```python
from build123d import *

# Parameters (mm, degrees)
F1_DEPTH = 25.4


with BuildPart() as f1:
    # F0 (on Top) → F1 (new body)
    with BuildSketch(Plane.XY):
        with BuildLine():
            ThreePointArc((0.5710253026, 3.1232283144), (0.8333744276, 3.0636762335), (1.0897403684, 2.9821285904))
            Line((1.0897403684, 2.9821285904), (1.0897403684, 10.6021285904))
            Line((1.0897403684, 10.6021285904), (0.5710253026, 10.6021285904))
            Line((0.5710253026, 10.6021285904), (0.5710253026, 3.1232283144))
        make_face()
        with BuildLine():
            ThreePointArc((-1.0897403684, 2.9821285904), (-0.8333744276, 3.0636762335), (-0.5710253026, 3.1232283144))
            Line((-0.5710253026, 3.1232283144), (-0.5710253026, 10.6021285904))
            Line((-0.5710253026, 10.6021285904), (-1.0897403684, 10.6021285904))
            Line((-1.0897403684, 10.6021285904), (-1.0897403684, 2.9821285904))
        make_face()
        with BuildLine():
            ThreePointArc((-2.9903077134, -1.0670917389), (-3.0699086609, -0.8101146916), (-3.1274693008, -0.5473214526))
            Line((-3.1274693008, -0.5473214526), (-9.7265828776, -4.3573214526))
            Line((-9.7265828776, -4.3573214526), (-9.4672253448, -4.8065418769))
            Line((-9.4672253448, -4.8065418769), (-2.9903077134, -1.0670917389))
        make_face()
        with BuildLine():
            Line((-8.6368425092, -6.2448071378), (-2.0377289324, -2.4348071378))
            ThreePointArc((-2.0377289324, -2.4348071378), (-2.2365342333, -2.2535615419), (-2.4192824108, -2.0561365755))
            Line((-2.4192824108, -2.0561365755), (-8.8962000421, -5.7955867135))
            Line((-8.8962000421, -5.7955867135), (-8.6368425092, -6.2448071378))
        make_face()
        with BuildLine():
            Line((8.8962000421, -5.7955867135), (2.4192824108, -2.0561365755))
            ThreePointArc((2.4192824108, -2.0561365755), (2.2365342333, -2.2535615419), (2.0377289324, -2.4348071378))
            Line((2.0377289324, -2.4348071378), (8.6368425092, -6.2448071378))
            Line((8.6368425092, -6.2448071378), (8.8962000421, -5.7955867135))
        make_face()
        with BuildLine():
            Line((9.7265828776, -4.3573214526), (3.1274693008, -0.5473214526))
            ThreePointArc((3.1274693008, -0.5473214526), (3.0699086609, -0.8101146916), (2.9903077134, -1.0670917389))
            Line((2.9903077134, -1.0670917389), (9.4672253448, -4.8065418769))
            Line((9.4672253448, -4.8065418769), (9.7265828776, -4.3573214526))
        make_face()
        with BuildLine():
            Line((0.5710253026, 2.9821285904), (1.0897403684, 2.9821285904))
            ThreePointArc((1.0897403684, 2.9821285904), (0.8333744276, 3.0636762335), (0.5710253026, 3.1232283144))
            Line((0.5710253026, 3.1232283144), (0.5710253026, 2.9821285904))
        make_face()
        with BuildLine():
            Line((-0.5710253026, 2.9821285904), (-0.5710253026, 3.1232283144))
            ThreePointArc((-0.5710253026, 3.1232283144), (-0.8333744276, 3.0636762335), (-1.0897403684, 2.9821285904))
            Line((-1.0897403684, 2.9821285904), (-0.5710253026, 2.9821285904))
        make_face()
        with BuildLine():
            ThreePointArc((3.1274693008, -0.5473214526), (3.1630950057, -0.2746907078), (3.175, 0))
            ThreePointArc((3.175, 0), (2.6019752756, 1.819436634), (1.0897403684, 2.9821285904))
            Line((1.0897403684, 2.9821285904), (0.5710253026, 2.9821285904))
            Line((0.5710253026, 2.9821285904), (-0.5710253026, 2.9821285904))
            Line((-0.5710253026, 2.9821285904), (-1.0897403684, 2.9821285904))
            ThreePointArc((-1.0897403684, 2.9821285904), (-2.749630657, 1.5875), (-3.1274693008, -0.5473214526))
            ThreePointArc((-3.1274693008, -0.5473214526), (-3.0699086609, -0.8101146916), (-2.9903077134, -1.0670917389))
            ThreePointArc((-2.9903077134, -1.0670917389), (-2.749630657, -1.5875), (-2.4192824108, -2.0561365755))
            ThreePointArc((-2.4192824108, -2.0561365755), (-2.2365342333, -2.2535615419), (-2.0377289324, -2.4348071378))
            ThreePointArc((-2.0377289324, -2.4348071378), (0, -3.175), (2.0377289324, -2.4348071378))
            ThreePointArc((2.0377289324, -2.4348071378), (2.2365342333, -2.2535615419), (2.4192824108, -2.0561365755))
            ThreePointArc((2.4192824108, -2.0561365755), (2.749630657, -1.5875), (2.9903077134, -1.0670917389))
            ThreePointArc((2.9903077134, -1.0670917389), (3.0699086609, -0.8101146916), (3.1274693008, -0.5473214526))
        make_face()
    extrude(amount=F1_DEPTH)


solid = f1.part
```
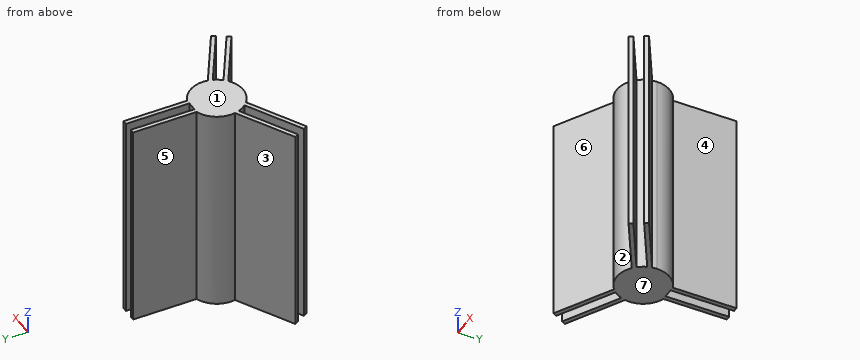
Design review of the part built by this model. Coordinates are the model's own, in mm. Face numbers are marked on the shaded views. A direction names the side the tool comes from. Coordinates: 2 decimals unless noted, no trailing zeros. Write each loop counter-clockwise with the first axis right and the second up, starting at its lowest first coordinate (ties: lowest second). Pieces come first, ordered by that corner, then holes. Notation, with made-up numbers: M 46.5,88.25 L 100.5,88.25 A25 cw 100.5,106.25 Z; hole C 36,83 d4. An arc over 180 degrees is marked long. Answer as a JSON object with one key per item and string values.
Item 1: Insertion check: pin 1 Ø1.5 at (y, z) = (-3.5, 4.5) entering from +X; pin 2 Ø6 at (y, z) = (8.5, 16) entering from +X; pin 3 Ø8 at (x, y) = (7.5, 5) entering from +Z; pin 4 Ø3 at (y, z) = (1, 17) entering from +X (3 decimals). Each pin has a flat end and moves straight along its axis. Give the tip position at first contact, or say it passes through.
Outcome:
{"pin 1": "x = 9.54", "pin 2": "x = 1.09", "pin 3": "through", "pin 4": "x = 3.175"}
Item 2: Add section B-B, the plane z = 19.5. Give the boundary of the cut face in (x, y) (3 decimals), and give its area (3 significant figures).
Outcome:
{"outline": "M -9.727,-4.357 L -9.467,-4.807 L -2.99,-1.067 A3.175 ccw -2.419,-2.056 L -8.896,-5.796 L -8.637,-6.245 L -2.038,-2.435 A3.175 ccw 2.038,-2.435 L 8.637,-6.245 L 8.896,-5.796 L 2.419,-2.056 A3.175 ccw 2.99,-1.067 L 9.467,-4.807 L 9.727,-4.357 L 3.127,-0.547 A3.175 ccw 1.09,2.982 L 1.09,10.602 L 0.571,10.602 L 0.571,2.982 L -0.571,2.982 L -0.571,10.602 L -1.09,10.602 L -1.09,2.982 A3.175 ccw -3.127,-0.547 Z", "area": "54.9 mm²"}
Item 3: Add section A-A, the plane y = 8. Give the boundary of the cut face in (x, z), and give its area (3 significant figures).
Outcome:
{"outline": "M -1.09,0 L -0.57,0 L -0.57,25.4 L -1.09,25.4 Z; M 0.57,0 L 1.09,0 L 1.09,25.4 L 0.57,25.4 Z", "area": "26.4 mm²"}
Item 4: Wall thickness on probe 1 along X at (y, z) = (8.5, 23.75); probe 2 along X at (y, z) = (-2.75, 18.5); probe 3 along X at (y, z) = (-4, 8.75): over which ranges is each line inside the solid? List them lowest first.
Outcome:
{"probe 1": "-1.09 to -0.57, 0.57 to 1.09", "probe 2": "-6.94 to -5.91, -3.62 to -2.58, -1.59 to 1.59, 2.58 to 3.62, 5.91 to 6.94", "probe 3": "-9.11 to -8.07, -5.79 to -4.75, 4.75 to 5.79, 8.07 to 9.11"}
Item 5: Add section C-C, the plane x = 6.75. Give the boundary of the cut face in (y, z).
Outcome:
{"outline": "M -5.16,0 L -4.56,0 L -4.56,25.4 L -5.16,25.4 Z; M -3.24,0 L -2.64,0 L -2.64,25.4 L -3.24,25.4 Z"}
Item 6: Machinability: for the marked faces 5, 6 and 7, which of the approach directions +Z, -Z, +X, -X, +Y, -Y give a long, thin tool a straight path to every point of the face, cutting with its end or side? Answer none if there is none.
Outcome:
{"face 5": "+Z, -Z, -X, +Y", "face 6": "+Z, -Z, -Y", "face 7": "-Z, +X, -X, +Y, -Y"}
Item 7: Draft analysis for pull direction X (two halves, no side actions). For the marked faces 1, 2, 3 and 4, state which applies: pulls with the +X half, pulls with the -X half, needs draft (parallel to the pull), parting line crosses it, or undercut.
Outcome:
{"face 1": "needs draft", "face 2": "undercut", "face 3": "pulls with the -X half", "face 4": "pulls with the +X half"}
